```python
from build123d import *

# Parameters (mm, degrees)
SKETCH_1_R               = 6
SKETCH_1_R_2             = 4
EXTRUDE_1_DEPTH          = 99
SKETCH_2_W               = 99
SKETCH_2_H               = 2
EXTRUDE_2_DEPTH          = 37
SKETCH_3_R               = 4
CUT_EXTRUDE_1_DEPTH      = 106.858395983
SKETCH_7_R               = 3.2
CUT_EXTRUDE_8_DEPTH      = 37
CUT_EXTRUDE_9_DEPTH      = 106.919780967
CUT_EXTRUDE_9_DEPTH_BACK = 106.919780967
SKETCH_8_W               = 21
SKETCH_8_H               = 14
SKETCH_8_W_2             = 27
CHAMFER_2_SIZE           = 1.5


with BuildPart() as part:
    # 草图1 → 凸台-拉伸1 (new body)
    with BuildSketch(Plane(origin=(0, 0, 0), x_dir=(0, 0, -1), z_dir=(1, 0, 0))):
        Circle(SKETCH_1_R)
        Circle(SKETCH_1_R_2, mode=Mode.SUBTRACT)
    extrude(amount=EXTRUDE_1_DEPTH)

    # 草图2 → 凸台-拉伸2 (add)
    with BuildSketch(Plane.XY):
        with Locations((49.5, -2)):
            Rectangle(SKETCH_2_W, SKETCH_2_H)
    extrude(amount=EXTRUDE_2_DEPTH)

    # 草图3 → 切除-拉伸1 (cut, through all)
    with BuildSketch(Plane.ZY):
        with Locations(Location((0, 0, 0), (0, 0, 180))):
            Circle(SKETCH_3_R)
    extrude(amount=-CUT_EXTRUDE_1_DEPTH, mode=Mode.SUBTRACT)

    # 草图7 → 切除-拉伸8 (cut)
    with BuildSketch(Plane.XZ.offset(3)):
        with Locations((12.5, 18)):
            Circle(SKETCH_7_R)
        with Locations((37, 27)):
            Circle(SKETCH_7_R)
        with Locations((62, 18)):
            Circle(SKETCH_7_R)
        with Locations((86.5, 27)):
            Circle(SKETCH_7_R)
    extrude(amount=-CUT_EXTRUDE_8_DEPTH, mode=Mode.SUBTRACT)

    # 草图8 → 切除-拉伸9 (cut, two sides: drawn at the far end of the back side and taken through both)
    with BuildSketch(Plane(origin=(0, -1, 0), x_dir=(1, 0, 0), z_dir=(0, 1, 0)).offset(-CUT_EXTRUDE_9_DEPTH_BACK)):
        with Locations((10.5, -1)):
            Rectangle(SKETCH_8_W, SKETCH_8_H)
        with Locations((49.5, -1)):
            Rectangle(SKETCH_8_W_2, SKETCH_8_H)
        with Locations((88.5, -1)):
            Rectangle(SKETCH_8_W, SKETCH_8_H)
    extrude(amount=CUT_EXTRUDE_9_DEPTH + CUT_EXTRUDE_9_DEPTH_BACK, mode=Mode.SUBTRACT)

    # 倒角2
    chamfer_2_edges = [part.edges().sort_by_distance(p)[0] for p in [
        (9.3, -1, 18),
        (33.8, -1, 27),
        (58.8, -1, 18),
        (83.3, -1, 27),
    ]]
    chamfer(chamfer_2_edges, length=CHAMFER_2_SIZE)


solid = part.part
```
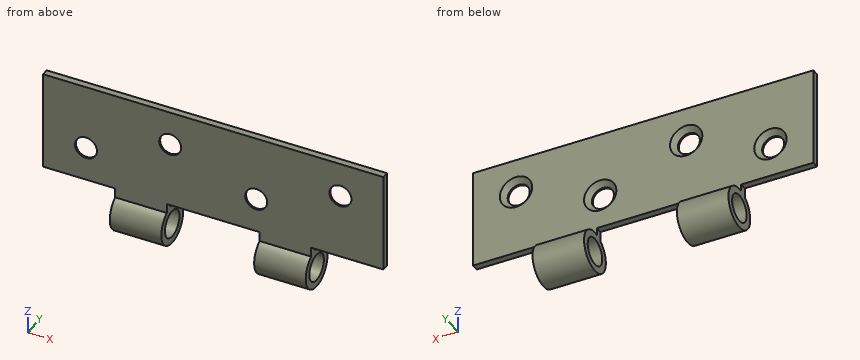
CAD build for the part. Positions are in the model's coordinates, mm. Round coordinates to 2 decimals unless told otherwise and drop trailing zeros. Order: outer loops, then holes, each group sorted by start corner. A loop starts at its lowest first (then second) coordinate and runs counter-clockwise, first axis right, second up. Notation, with made-up numbers: (-17.75, -26) - (40.25, -26) arc R24 ccw to (40.25, -5) - close; hole circle Ø10 at (35.5, -0.5). An arc over 180 degrees is marked (long way). Use CSV: the item, a comma, the result in double quotes. Start each with the question number.
1) Saw through at A-A (z = 0). List the corners of the cut face in (x, y), and give its area (3 significant figures).
2) Wall check: L1, parallel to X at y = -1.5, z = 28.5; L2, parallel to Z at x = 86.5, y = -2.8; L3, parallel to Y at x = 30.25, z = 0. Give the ranges that are in metal, low to high. Write a range as [from, to].
3) Pin check, flat tips, straight feed: pin 1 Ø2 at (x, y) = (6, -2) entering from -Z; pin 2 Ø1.5 at (x, z) = (88.5, 23.5) entering from +Y; pin 3 Ø4 at (x, y) = (63.5, 4.5) entering from -Z. Stop position of each tip, or through.
4) Saw through at B-B (x = 86.5). List the corners of the cut face in (y, z), and give its area (4 significant figures).
5) Saw through at C-C (z = 18). List the corners of the cut face in (x, y).
6) Saw through at D-D (y = 1.75). List the corners of the cut face in (x, z).
Values follow:
1,outline,"(21, -6) - (36, -6) - (36, -4) - (21, -4) - close; (21, 4) - (36, 4) - (36, 6) - (21, 6) - close; (63, -6) - (78, -6) - (78, -4) - (63, -4) - close; (63, 4) - (78, 4) - (78, 6) - (63, 6) - close"
1,area,"120 mm2"
2,L1,"x = [0, 33.08], [40.92, 82.58], [90.42, 99]"
2,L2,"z = [8, 23.8], [30.2, 37]"
2,L3,"y = [-6, -4], [4, 6]"
3,pin 1,"stops at z = 8"
3,pin 2,"stops at y = -1"
3,pin 3,"stops at z = -5.45"
4,outline,"(-3, 8) - (-1, 8) - (-1, 22.3) - (-2.5, 23.8) - (-3, 23.8) - close; (-3, 30.2) - (-2.5, 30.2) - (-1, 31.7) - (-1, 37) - (-3, 37) - close"
4,area,"42.95 mm2"
5,outline,"(0, -3) - (9.3, -3) - (9.3, -2.5) - (7.8, -1) - (0, -1) - close; (15.7, -3) - (58.8, -3) - (58.8, -2.5) - (57.3, -1) - (17.2, -1) - (15.7, -2.5) - close; (65.2, -3) - (99, -3) - (99, -1) - (66.7, -1) - (65.2, -2.5) - close"
6,outline,"(21, -5.74) - (36, -5.74) - (36, -3.6) - (21, -3.6) - close; (21, 3.6) - (36, 3.6) - (36, 5.74) - (21, 5.74) - close; (63, -5.74) - (78, -5.74) - (78, -3.6) - (63, -3.6) - close; (63, 3.6) - (78, 3.6) - (78, 5.74) - (63, 5.74) - close"
